Build history of the part. All positions in model axes, mm. Face numbers are marked on the shaded views. A direction names the side the tool comes from. Round coordinates to 2 decimals unless told otherwise and drop trailing zeros. Write each loop counter-clockwise with the first axis right and the second up, starting at its lowest first coordinate (ties: lowest second). Pieces come first, ordered by that corner, then holes. Notation, with made-up numbers: (79.5, 89.5) - (135.5, 89.5) arc R16 ccw to (135.5, 95.5) - close; hole circle Ø8 at (29.5, 36.5). An arc over 180 degrees is marked (long way). Write each question's results on one line, items separated by ' | '.
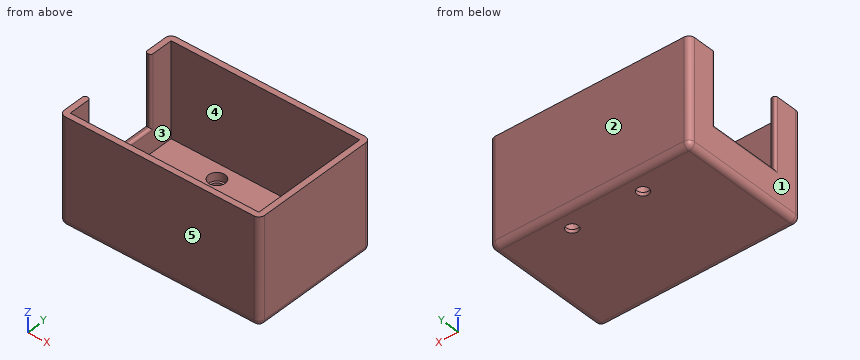
Autodesk Fusion 360 part; units mm, degrees
sketch "Sketch1" plane through (0, 0, 0) normal (0, 0, 1) x (1, 0, 0)
  line L0 (0, 0) -> (160, 0)
  line L1 (160, 0) -> (160, 100)
  line L2 (160, 100) -> (0, 100)
  line L3 (0, 100) -> (0, 0)
  line L4 (-5, -5) -> (165, -5)
  line L5 (165, -5) -> (165, 105)
  line L6 (165, 105) -> (-5, 105)
  line L7 (-5, 105) -> (-5, -5)
  circle A0 centre (50, 87) radius 5
  circle A1 centre (50, 87) radius 7
  circle A2 centre (110, 87) radius 5
  circle A3 centre (110, 87) radius 7
  dimension "d1" = 160
  dimension "d2" = 100
  dimension "d3" = 14
  dimension "d4" = 10
  dimension "d5" = 14
extrude "Extrude1" add sketch "Sketch1" along normal blind 3 contours A1 makes body 1
extrude "Extrude2" add sketch "Sketch1" along normal blind 3 separate body contours A3 makes body 2
extrude "Extrude3" add sketch "Sketch1" along normal blind 10 contours L0 L1 L2 L3 bodies 1 2
extrude "Extrude4" add sketch "Sketch1" along normal blind 90 contours L4 L5 L6 L7 bodies 1
sketch "Sketch2" plane through (0, 0, 90) normal (0, 0, 1) x (-1, 0, 0)
  line L0 (0, 0) -> (0, -100)
  line L1 (0, -100) -> (-160, -100)
  line L2 (-160, -100) -> (-160, 0)
  line L3 (-160, 0) -> (0, 0)
  line L4 (5, -105) -> (5, 5)
  line L5 (5, 5) -> (-165, 5)
  line L6 (-165, 5) -> (-165, -105)
  line L7 (-165, -105) -> (5, -105)
  line L8 (5, -80) -> (0, -80)
  line L9 (0, -80) -> (0, -20)
  line L10 (0, -20) -> (5, -20)
  line L11 (5, -20) -> (5, -80)
extrude "Extrude5" cut sketch "Sketch2" against normal blind 60 contours L0 L4 L8 L9 L10 L11 bodies 1
fillet "Fillet1" radius 5 8 edges at (-5, -5, 45) (-5, 50, 0) (80, -5, 0) (165, -5, 45) (165, 50, 0) (165, 105, 45) (80, 105, 0) (-5, 105, 45) on bodies 1
fillet "Fillet1" radius 2 6 edges at (-5, 80, 60) (0, 80, 60) (-5, 20, 60) (0, 20, 60) (-5, 50, 30) (0, 50, 30) on bodies 1
(1) Tool access for the marked faces 4 and 5: list every direction of +Z, -Z, +X, -X, +Y, -Y with a clear straight run to the whole face (end or side of a thin tool).
Worked answers:
face 4: +Z | face 5: +Z, -Z, +X, -X, -Y
(2) Flat gauge pins, fed straight in: pin 1 Ø4 at (x, y) = (113.5, 87.5) entering from +Z; pin 2 Ø0.5 at (x, y) = (-2.5, 49.5) entering from +Z; pin 3 Ø0.8 at (x, z) = (-2.5, 74) entering from -Y. Where does each tip first touch, or does it go through?
Worked answers:
pin 1: stops at z = 3 | pin 2: stops at z = 30 | pin 3: stops at y = -4.54
(3) Drill centre lines: probe 1 along Y at (x, z) = (43, 23); probe 2 along Y at (x, z) = (50, 4.5); probe 3 along X at (y, z) = (6.5, 70). Where is each one in solid material? Low to high. Write a range as [from, to].
Worked answers:
probe 1: y = [-5, 0], [100, 105] | probe 2: y = [-4.97, 80], [94, 104.97] | probe 3: x = [-5, 0], [160, 165]
(4) Two-plate mould, pull along X, no slides. Class the marked faces 1, 2 and 3: released by +X, released by -X, zero draft, split by the parting line, or undercut.
Worked answers:
face 1: released by -X | face 2: zero draft | face 3: undercut
(5) Slice it at B-B, the plane x = 110. Write the cut outline in (y, z), and give its area (3 significant figures).
Worked answers:
outline: (-5, 5) arc R5 ccw to (0, 0) - (82, 0) - (82, 3) - (80, 3) - (80, 10) - (0, 10) - (0, 90) - (-5, 90) - close; (92, 0) - (100, 0) arc R5 ccw to (105, 5) - (105, 90) - (100, 90) - (100, 10) - (94, 10) - (94, 3) - (92, 3) - close | area: 1,760 mm2
(6) Slice it at A-A, the plane z = 7.5. Write the cut outline in (x, y).
Worked answers:
outline: (-5, 0) arc R5 ccw to (0, -5) - (160, -5) arc R5 ccw to (165, 0) - (165, 100) arc R5 ccw to (160, 105) - (0, 105) arc R5 ccw to (-5, 100) - close; hole circle Ø14 at (50, 87); hole circle Ø14 at (110, 87)
(7) Slice it at D-D, the plane y = 47.5. Write the cut outline in (x, z), and give its area (3 significant figures).
Worked answers:
outline: (-5, 5) arc R5 ccw to (0, 0) - (160, 0) arc R5 ccw to (165, 5) - (165, 90) - (160, 90) - (160, 10) - (0, 10) - (0, 28) arc R2 ccw to (-2, 30) - (-3, 30) arc R2 ccw to (-5, 28) - close | area: 2,190 mm2
(8) Slice it at C-C, the plane z = 20.5. Write the cut outline in (x, y), and give its area (3 significant figures).
Worked answers:
outline: (-5, 0) arc R5 ccw to (0, -5) - (160, -5) arc R5 ccw to (165, 0) - (165, 100) arc R5 ccw to (160, 105) - (0, 105) arc R5 ccw to (-5, 100) - close; hole (0, 0) - (160, 0) - (160, 100) - (0, 100) - close | area: 2,680 mm2
